from build123d import *

# Parameters (mm, degrees)
SKETCH1_R           = 20.9
BOSS_EXTRUDE1_DEPTH = 30
SKETCH2_R           = 1
CUT_EXTRUDE1_DEPTH  = 3
SKETCH3_R           = 1
CUT_EXTRUDE2_DEPTH  = 3
SKETCH6_R           = 22.9
SKETCH6_R_2         = 18.4
BOSS_EXTRUDE2_DEPTH = 12
FILLET1_R           = 10
CHAMFER1_SIZE       = 2
SKETCH4_W           = 15
SKETCH4_H           = 3.988700157
CUT_EXTRUDE3_DEPTH  = 83.82344173
SKETCH8_R           = 1
CUT_EXTRUDE4_DEPTH  = 2
FILLET2_R           = 3
FILLET3_R           = 3
SKETCH9_W           = 164.009429166
SKETCH9_H           = 28.275732928
CUT_EXTRUDE5_DEPTH  = 93


with BuildPart() as part:
    # Sketch1 → Boss-Extrude1 (new body)
    with BuildSketch(Plane(origin=(0, 0, 0), x_dir=(1, 0, 0), z_dir=(0, 1, 0))):
        with BuildLine():
            Line((-41.094820281, 6.777775896), (-45, -16.9))
            Line((-45, -16.9), (-65, -16.9))
            Line((-65, -16.9), (-65, -36.9))
            Line((-65, -36.9), (65, -36.9))
            Line((65, -36.9), (65, -16.9))
            Line((65, -16.9), (45, -16.9))
            Line((45, -16.9), (41.094820281, 6.777775896))
            ThreePointArc((41.094820281, 6.777775896), (0, 41.65), (-41.094820281, 6.777775896))
        make_face()
        with Locations(Location((0, 0, 0), (0, 0, 270))):
            Circle(SKETCH1_R, mode=Mode.SUBTRACT)
    extrude(amount=BOSS_EXTRUDE1_DEPTH)

    # Sketch2 → Cut-Extrude1 (cut)
    with BuildSketch(Plane(origin=(0, 0, 16.9), x_dir=(-1, 0, 0), z_dir=(0, 0, -1))):
        with Locations((-55, 15)):
            Circle(SKETCH2_R)
    extrude(amount=-CUT_EXTRUDE1_DEPTH, mode=Mode.SUBTRACT)

    # Sketch3 → Cut-Extrude2 (cut)
    with BuildSketch(Plane(origin=(0, 0, 16.9), x_dir=(-1, 0, 0), z_dir=(0, 0, -1))):
        with Locations((55, 15)):
            Circle(SKETCH3_R)
    extrude(amount=-CUT_EXTRUDE2_DEPTH, mode=Mode.SUBTRACT)

    # Sketch6 → Boss-Extrude2 (add)
    with BuildSketch(Plane.XZ):
        Circle(SKETCH6_R)
        with Locations(Location((0, 0, 0), (0, 0, 270))):
            Circle(SKETCH6_R_2, mode=Mode.SUBTRACT)
    extrude(amount=-BOSS_EXTRUDE2_DEPTH)

    # Fillet1
    fillet1_edges = [part.edges().sort_by_distance(p)[0] for p in [
        (-45, 15, 16.9),
        (45, 15, 16.9),
    ]]
    fillet(fillet1_edges, radius=FILLET1_R)

    # Chamfer1
    chamfer1_edges = [part.edges().sort_by_distance(p)[0] for p in [
        (0, 30, -20.9),
    ]]
    chamfer(chamfer1_edges, length=CHAMFER1_SIZE)

    # Sketch4 → Cut-Extrude3 (cut, through all)
    with BuildSketch(Plane.XZ):
        with Locations((0, -42.963515313)):
            Rectangle(SKETCH4_W, SKETCH4_H)
    extrude(amount=-CUT_EXTRUDE3_DEPTH, mode=Mode.SUBTRACT)

    # Sketch8 → Cut-Extrude4 (cut)
    with BuildSketch(Plane(origin=(0, 0, -40.969165234), x_dir=(-1, 0, 0), z_dir=(0, 0, -1))):
        with Locations((0, 22)):
            Circle(SKETCH8_R)
    extrude(amount=-CUT_EXTRUDE4_DEPTH, mode=Mode.SUBTRACT)

    # Fillet2
    # the kernel refuses this fillet: 3 mm, written as the material it takes off along each edge
    with BuildSketch(Plane(origin=(83, 30, 16.9), x_dir=(0, 0, 1), z_dir=(-1, 0, 0)), Plane(origin=(-53.485795501, 30, 16.9), x_dir=(0, 0, 1), z_dir=(-1, 0, 0))) as fillet2_piece_1:
        with BuildLine():
            CenterArc((FILLET2_R, -FILLET2_R), FILLET2_R, 90, 90)
            Line((0, -FILLET2_R), (-FILLET2_R * 0.02, -FILLET2_R))
            Line((-FILLET2_R * 0.02, -FILLET2_R), (-FILLET2_R * 0.02, FILLET2_R * 0.02))
            Line((-FILLET2_R * 0.02, FILLET2_R * 0.02), (FILLET2_R, FILLET2_R * 0.02))
            Line((FILLET2_R, FILLET2_R * 0.02), (FILLET2_R, 0))
        make_face()
    extrude(amount=29.514204499, mode=Mode.SUBTRACT)
    with BuildSketch(Plane(origin=(53.485795501, 30, 6.9), x_dir=(-0.9866703548806417, 0, 0.1627317141792235), z_dir=(-0.1627317141792235, 0, -0.9866703548806417))) as fillet2_piece_2:
        with BuildLine():
            CenterArc((10 + FILLET2_R, -FILLET2_R), FILLET2_R, 90, 90)
            Line((10, -FILLET2_R), (10 - FILLET2_R * 0.02, -FILLET2_R))
            Line((10 - FILLET2_R * 0.02, -FILLET2_R), (10 - FILLET2_R * 0.02, FILLET2_R * 0.02))
            Line((10 - FILLET2_R * 0.02, FILLET2_R * 0.02), (10 + FILLET2_R, FILLET2_R * 0.02))
            Line((10 + FILLET2_R, FILLET2_R * 0.02), (10 + FILLET2_R, 0))
        make_face()
    revolve(axis=Axis((53.485795501, 30, 6.9), (0, 1, 0)), revolution_arc=80.6345096, mode=Mode.SUBTRACT)
    with BuildSketch(Plane(origin=(43.619091952, 30, 8.527317142), x_dir=(-0.9866703548806418, 0, 0.16273171417922358), z_dir=(-0.16273171417922358, 0, -0.9866703548806418)), Plane(origin=(-41.094820281, 30, -6.777775896), x_dir=(0.9866703548806418, 0, 0.16273171417922358), z_dir=(-0.16273171417922358, 0, 0.9866703548806418))) as fillet2_piece_3:
        with BuildLine():
            CenterArc((FILLET2_R, -FILLET2_R), FILLET2_R, 90, 90)
            Line((0, -FILLET2_R), (-FILLET2_R * 0.02, -FILLET2_R))
            Line((-FILLET2_R * 0.02, -FILLET2_R), (-FILLET2_R * 0.02, FILLET2_R * 0.02))
            Line((-FILLET2_R * 0.02, FILLET2_R * 0.02), (FILLET2_R, FILLET2_R * 0.02))
            Line((FILLET2_R, FILLET2_R * 0.02), (FILLET2_R, 0))
        make_face()
    extrude(amount=15.511860635, mode=Mode.SUBTRACT)
    with BuildSketch(Plane(origin=(-53.485795501, 30, 6.9), x_dir=(0.9866703548806417, 0, 0.1627317141792235), z_dir=(0.1627317141792235, 0, -0.9866703548806417))) as fillet2_piece_4:
        with BuildLine():
            CenterArc((10 + FILLET2_R, FILLET2_R), FILLET2_R, 180, 90)
            Line((10, FILLET2_R), (10 - FILLET2_R * 0.02, FILLET2_R))
            Line((10 - FILLET2_R * 0.02, FILLET2_R), (10 - FILLET2_R * 0.02, -FILLET2_R * 0.02))
            Line((10 - FILLET2_R * 0.02, -FILLET2_R * 0.02), (10 + FILLET2_R, -FILLET2_R * 0.02))
            Line((10 + FILLET2_R, -FILLET2_R * 0.02), (10 + FILLET2_R, 0))
        make_face()
    revolve(axis=Axis((-53.485795501, 30, 6.9), (0, -1, 0)), revolution_arc=80.6345096, mode=Mode.SUBTRACT)
    with BuildSketch(Plane(origin=(0, 30, 0), x_dir=(0.24858486581871286, 0, -0.9686101199584343), z_dir=(0.9686101199584343, 0, 0.24858486581871286))) as fillet2_piece_5:
        with BuildLine():
            CenterArc((41.65 - FILLET2_R, -FILLET2_R), FILLET2_R, 0, 90)
            Line((41.65, -FILLET2_R), (41.65 + FILLET2_R * 0.02, -FILLET2_R))
            Line((41.65 + FILLET2_R * 0.02, -FILLET2_R), (41.65 + FILLET2_R * 0.02, FILLET2_R * 0.02))
            Line((41.65 + FILLET2_R * 0.02, FILLET2_R * 0.02), (41.65 - FILLET2_R, FILLET2_R * 0.02))
            Line((41.65 - FILLET2_R, FILLET2_R * 0.02), (41.65 - FILLET2_R, 0))
        make_face()
    revolve(axis=Axis((0, 30, 0), (0, 1, 0)), revolution_arc=95.028297231, mode=Mode.SUBTRACT)
    with BuildSketch(Plane(origin=(0, 30, 0), x_dir=(0.9866703548806417, 0, -0.16273171417922386), z_dir=(0.16273171417922386, 0, 0.9866703548806417))) as fillet2_piece_6:
        with BuildLine():
            CenterArc((41.65 - FILLET2_R, -FILLET2_R), FILLET2_R, 0, 90)
            Line((41.65, -FILLET2_R), (41.65 + FILLET2_R * 0.02, -FILLET2_R))
            Line((41.65 + FILLET2_R * 0.02, -FILLET2_R), (41.65 + FILLET2_R * 0.02, FILLET2_R * 0.02))
            Line((41.65 + FILLET2_R * 0.02, FILLET2_R * 0.02), (41.65 - FILLET2_R, FILLET2_R * 0.02))
            Line((41.65 - FILLET2_R, FILLET2_R * 0.02), (41.65 - FILLET2_R, 0))
        make_face()
    revolve(axis=Axis((0, 30, 0), (0, 1, 0)), revolution_arc=95.028297231, mode=Mode.SUBTRACT)

    # Fillet3
    fillet3_edges = [part.edges().sort_by_distance(p)[0] for p in [
        (65, 30, 28.4),
        (-65, 30, 28.4),
        (65, 13.5, 16.9),
        (65, 29.121320344, 17.778679656),
        (-65, 13.5, 16.9),
        (-65, 29.121320344, 17.778679656),
    ]]
    fillet(fillet3_edges, radius=FILLET3_R)

    # Sketch9 → Cut-Extrude5 (cut)
    with BuildSketch(Plane.XY.offset(36.9)):
        with Locations((5.097067232, 20.137866464)):
            Rectangle(SKETCH9_W, SKETCH9_H)
    extrude(amount=-CUT_EXTRUDE5_DEPTH, mode=Mode.SUBTRACT)


solid = part.part
For this review, take the finished solid that the model builds, in its own axes (mm). A direction names the side the tool comes from. Round coordinates to 2 decimals unless told otherwise and drop trailing zeros. Write each loop counter-clockwise with the first axis right and the second up, starting at its lowest first coordinate (ties: lowest second). Pieces come first, ordered by that corner, then holes. Notation, with made-up numbers: (6.5, 69.5) - (60.5, 69.5) arc R17 cw to (60.5, 85.5) - close; hole circle Ø7 at (23, 87.5). An arc over 180 degrees is marked (long way). Write item = value, one per line. Start each with the question number.
1. For faces 1 (the face through (-1, 3, 36.9)), 2 (the face through (-58, 3, 16.9)), 3 (the face through (58, 3, 16.9)), list the 3-axis set-ups (+Z, -Z, +X, -X, +Y, -Y) from which the entire face can be reached by the end or side of a thin tool; tool diameter is ignored.
2. Draft analysis for pull direction Z (two halves, no side actions). For faces 4 (the face through (46.94, 3.04, 14.46)), 5 (the face through (5.53, 2.96, -17.55)), 6 (the face through (65, 3, 29)), state which applies: released by +Z, released by -Z, zero draft, split by the parting line, or undercut.
3. Wall thickness on L1, parallel to Z at x = -1, y = 3.35; L2, parallel to X at y = 2.2, z = 0; L3, parallel to Z at x = 8, y = 4.1: over which ranges is each line inside the solid? List them lowest first.
4. Consider section C-C on z = 0. State the section outline as (x, y) points.
5. For pin 1 Ø3 at (x, z) = (-25.5, 4.5) entering from -Y; pin 2 Ø3 at (x, y) = (59, 3.5) entering from -Z, all flat-tipped, find the tip position at first contact; note any pin that passes through.
6. Consider section A-A on x = 0. State the section outline as (y, z) points.
7. Consider section D-D on z = -20.5. State the section outline as (x, y) points.
8. Consider section B-B on y = 1.75. State the section outline as (x, z) points, plus the area to 3 significant figures.
Evaluation:
q1.face_1 = +Z, +X, -X, +Y, -Y
q1.face_2 = -Z, -X, +Y, -Y
q1.face_3 = -Z, +X, +Y, -Y
q2.face_4 = released by -Z
q2.face_5 = undercut
q2.face_6 = zero draft
q3.L1 = -40.97 to -18.37, 18.37 to 36.9
q3.L2 = -42.21 to -18.4, 18.4 to 42.21
q3.L3 = -40.87 to -16.57, 16.57 to 36.9
q4.outline = (-42.21, 0) - (-18.4, 0) - (-18.4, 6) - (-42.21, 6) - close; (18.4, 0) - (42.21, 0) - (42.21, 6) - (18.4, 6) - close
q5.pin_1 = 0
q5.pin_2 = 16.9
q6.outline = (0, -40.97) - (6, -40.97) - (6, -18.4) - (0, -18.4) - close; (0, 18.4) - (6, 18.4) - (6, 36.9) - (0, 36.9) - close
q7.outline = (-36.26, 0) - (36.26, 0) - (36.26, 6) - (-36.26, 6) - close
q8.outline = (-65, 19.9) arc R3 ccw to (-62, 16.9) - (-53.49, 16.9) arc R10 cw to (-43.62, 8.53) - (-41.09, -6.78) arc R41.65 ccw to (-7.5, -40.97) - (7.5, -40.97) arc R41.65 ccw to (41.09, -6.78) - (43.62, 8.53) arc R10 cw to (53.49, 16.9) - (62, 16.9) arc R3 ccw to (65, 19.9) - (65, 36.9) - (-65, 36.9) - close; hole circle Ø36.8 at (0, 0)
q8.area = 5,760 mm2
